Check sheet for the drawn part. Datum: minimum x, y, z corner. Units: mm. Round coordinates to 2 decimals unless told otherwise and drop trailing zeros. Write each loop counter-clockwise with the first axis right and the second up, starting at its lowest first coordinate (ties: lowest second). Pieces come first, ordered by that corner, then holes.
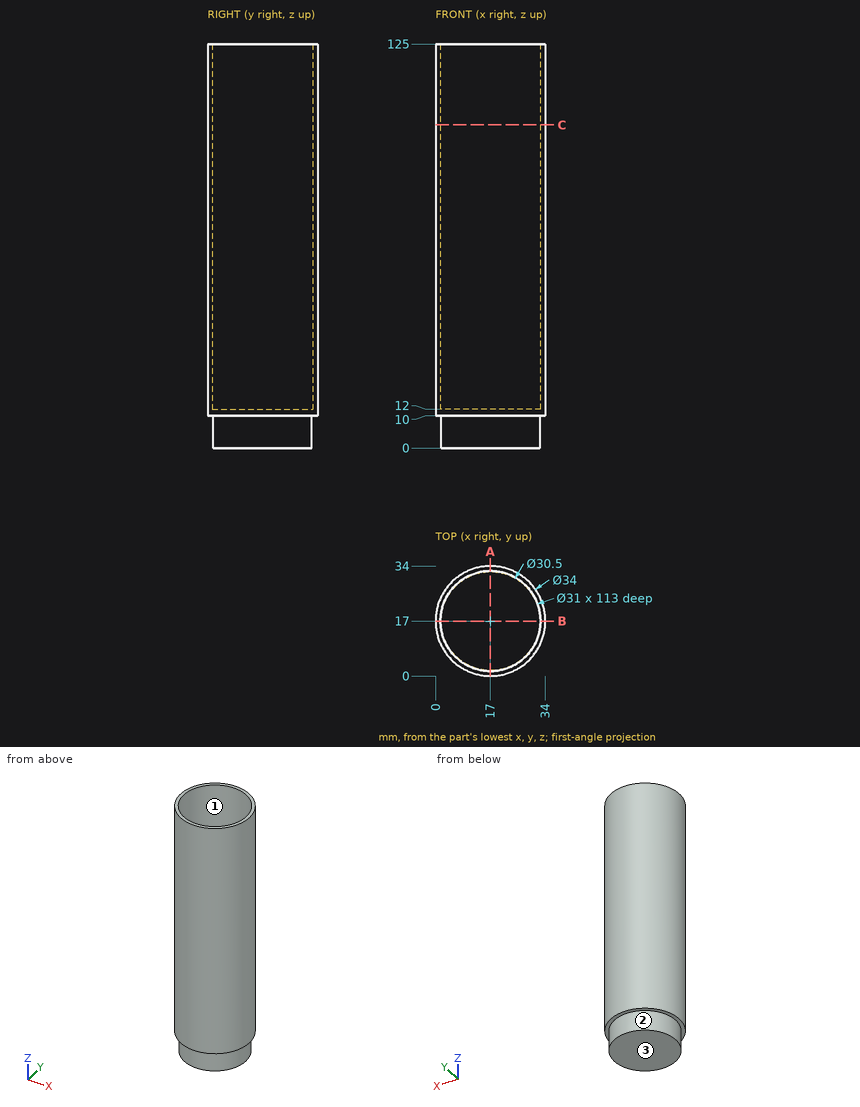
1. Release check for a two-part mould opening along X. For the marked faces 1, 2 and 3 record: released by +X, released by -X, zero draft, split by the parting line, or undercut.
2. Go/stop test with flat-tipped pins: pin 1 (1 mm diameter, centred on x = 29, z = 21, fed in from +Y); pin 2 (4 mm diameter, centred on x = 25.5, z = 63, fed in from -Y); pin 3 (6 mm diameter, centred on y = 29, z = 98, fed in from -X); pin 4 (12 mm diameter, centred on x = 20.5, z = 66, fed in from +Y). Record where each tip stops, or that it passes through.
3. Sectioned sample at C-C, the plane z = 100. Enter the section's corners in (x, y).
4. Scan lines: line 1 along Y through (x, z) = (17, 83); line 2 along Z through (x, y) = (12, 18.5); line 3 along Y through (x, z) = (30, 95). Record each from-to range of solid material in increasing order.
5. Sectioned sample at A-A, the plane x = 17. Enter the section's corners in (y, z), plus the area to 3 significant figures.
Computed values:
1. face 1: undercut
1. face 2: split by the parting line
1. face 3: zero draft
2. pin 1: stops at y = 29.52
2. pin 2: stops at y = 1.29
2. pin 3: stops at x = 2.58
2. pin 4: stops at y = 34
3. outline: circle Ø34 at (17, 17); hole circle Ø31 at (17, 17)
4. line 1: y = 0 to 1.5, 32.5 to 34
4. line 2: z = 0 to 12
4. line 3: y = 6.05 to 8.56, 25.44 to 27.95
5. outline: (0, 10) - (1.75, 10) - (1.75, 0) - (32.25, 0) - (32.25, 10) - (34, 10) - (34, 125) - (32.5, 125) - (32.5, 12) - (1.5, 12) - (1.5, 125) - (0, 125) - close
5. area: 712 mm2
